Answer from the drawing. Dimensions are ordinates in mm from the lowest x, y and z of the part. A direction names the side the tool comes from. Coordinates: 2 decimals unless noted, no trailing zeros. Write each loop counter-clockwise with the first axis right and the second up, starting at its lowest first coordinate (ties: lowest second). Pieces come first, ordered by that corner, then holes.
1) Which of the six approach directions +Z, -Z, +X, -X, +Y, -Y give full straight-line access (tool end or side, diameter ignored) to the marked faces 1, 2, 3 and 4?
2) The part is cut by section A-A (z = 8). Determine the outline of the cut face in (x, y) (3 decimals).
3) The part is cut by section D-D (y = 21). Determine the outline of the cut face in (x, z) (3 decimals).
4) The part is cut by section B-B (x = 12.85). Determine the outline of the cut face in (y, z), then the cut area to 3 significant figures.
5) Each of these flat-tipped pins is pushed along its axis until it touches: pin 1 Ø1.5 at (y, z) = (5, 7.5) entering from +X (3 decimals); pin 2 Ø4 at (y, z) = (12.5, 7) entering from +X; pin 3 Ø2.5 at (y, z) = (4.5, 6.5) entering from -X (3 decimals). Where does it stop, or does it pass through?
6) Find the intervals of material crossed by line 1 (Z direction, x = 6.5, y = 14); line 2 (X direction, y = 21, z = 8.75) (3 decimals); line 3 (X direction, y = 14.5, z = 8), in increasing order.
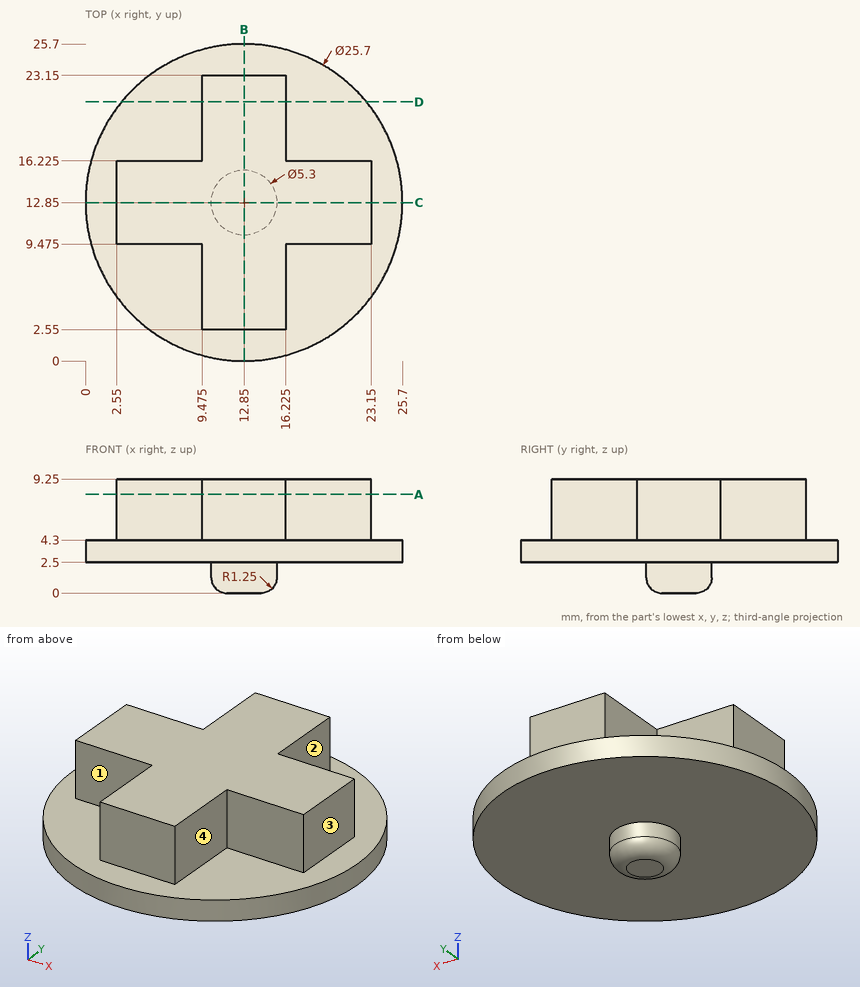
Reported:
1. face 1: +Z, -X, -Y
1. face 2: +Z, +X, +Y
1. face 3: +Z, +X, +Y, -Y
1. face 4: +Z, +X, -Y
2. outline: (2.55, 9.475) - (9.475, 9.475) - (9.475, 2.55) - (16.225, 2.55) - (16.225, 9.475) - (23.15, 9.475) - (23.15, 16.225) - (16.225, 16.225) - (16.225, 23.15) - (9.475, 23.15) - (9.475, 16.225) - (2.55, 16.225) - close
3. outline: (2.915, 2.5) - (22.785, 2.5) - (22.785, 4.3) - (16.225, 4.3) - (16.225, 9.25) - (9.475, 9.25) - (9.475, 4.3) - (2.915, 4.3) - close
4. outline: (0, 2.5) - (10.2, 2.5) - (10.2, 1.25) arc R1.25 ccw to (11.45, 0) - (14.25, 0) arc R1.25 ccw to (15.5, 1.25) - (15.5, 2.5) - (25.7, 2.5) - (25.7, 4.3) - (23.15, 4.3) - (23.15, 9.25) - (2.55, 9.25) - (2.55, 4.3) - (0, 4.3) - close
4. area: 161 mm2
5. pin 1: stops at x = 16.225
5. pin 2: stops at x = 23.15
5. pin 3: stops at x = 9.475
6. line 1: z = 2.5 to 9.25
6. line 2: x = 9.475 to 16.225
6. line 3: x = 2.55 to 23.15
